For this review, take the finished solid that the model builds, in its own axes (mm). A direction names the side the tool comes from. Give positions to 0.01 mm unless a question says otherwise; leave off trailing zeros. Order: outer loops, then holes, each group sorted by start corner. A loop starts at its lowest first (then second) coordinate and runs counter-clockwise, first axis right, second up. Notation, with made-up numbers: (18.25, 63.5) - (41.25, 63.5) arc R15 ccw to (41.25, 86.5) - close; hole circle Ø1 at (63, -18.75). An arc over 180 degrees is marked (long way). Use a Markdown table: item, result. Add a question column.
1) We need section A-A on y = 5.5. Write out the cut boundary in (x, z), then the cut area to 3 significant figures.
2) We need section D-D on x = 15.25. Give the number of separate pieces and of enclosed holes in the cut face, then the cut area to 3 significant figures.
3) Wall thickness on L1, parallel to Z at x = 2, y = -13.5; L2, parallel to X at y = 27, z = -15; L3, parallel to Y at x = 18.25, z = -12.5: over which ranges is each line inside the solid? List them lowest first.
4) Machinability: for faces 1 (the face through (20, -7.25, -11)), 2 (the face through (17, 0, -1)), 3 (the face through (23, 26, -12.95)), which of the approach directions +Z, -Z, +X, -X, +Y, -Y give a long, thin tool a straight path to every point of the face, cutting with its end or side? Answer none if there is none.
5) Mouldability with a two-part tool opening along Y and no side actions: class faces 4 (the face through (20, -6, -13.6)), 5 (the face through (20, -4.25, -11)), 6 (the face through (9.367, 35.797, -1.141)), 7 (the face through (9.63, 5.95, -21.13)) as released by +Y, released by -Y, zero draft, split by the parting line, or undercut.
6) We need section C-C on y = 26. Write out the cut boundary in (x, z), then the cut area to 3 significant figures.
7) Clearance check with flat-ended pins moving along their axes: P1, Ø5, axis at y = 23.5, z = -19.5, coming from the -X side; P2, Ø2, axis at x = 20.5, z = -10, coming from the -Y side; P3, Ø6, axis at y = -7.5, z = -9.5, coming from the +X side. State where each tip first meets the part, or that it passes through.
8) We need section B-B on z = -7.75. Write out the cut boundary in (x, y).
Autodesk Inventor part; units mm, degrees
ref_plane "YZ Plane" through (0, 0, 0) normal (1, 0, 0) x (0, 1, 0)
ref_plane "XZ Plane" through (0, 0, 0) normal (0, 1, 0) x (-1, 0, 0)
ref_plane "XY Plane" through (0, 0, 0) normal (0, 0, 1) x (1, 0, 0)
sketch "Sketch1" plane through (0, 0, 0) normal (1, 0, 0) x (0, 1, 0)
  line L0 (0, 0) -> (33, 0)
  line L1 (37, -4) -> (37, -18.2)
  line L2 (33, -22.2) -> (0, -22.2)
  line L3 (0, -22.2) -> (0, 0)
  arc A0 (33, -22.2) -> (37, -18.2) centre (33, -18.2) ccw
  arc A1 (37, -4) -> (33, 0) centre (33, -4) ccw
extrude "Extrusion1" add sketch "Sketch1" along normal blind 19
sketch "Sketch2" plane through (19, 0, 0) normal (1, 0, 0) x (0, 0, -1)
  line L0 (0, 33) -> (0, 0)
  line L1 (22.2, 37) -> (0, 37)
  line L2 (0, 37) -> (0, 26)
  line L3 (22.2, 26) -> (22.2, 37)
  line L4 (0, 31.5) -> (0, 26)
  circle A0 centre (11.1, 26) radius 2.65
  dimension "d9" = 11
  dimension "d11" = 5.3
extrude "Extrusion2" add sketch "Sketch2" along normal blind 8
sketch "Sketch3" plane through (27, 26, -11.1) normal (1, 0, 0) x (0, 0, -1)
  line L0 (1.85, 0) -> (1.85, -3.8405)
  line L1 (1.85, -3.8405) -> (0, -3.8405)
  line L2 (1.85, -3.8405) -> (-1.85, -3.8405)
  line L3 (-1.85, -3.8405) -> (-1.85, 4.0175)
  line L4 (-1.85, 4.0175) -> (1.85, 4.0175)
  line L5 (1.85, 4.0175) -> (1.85, -3.8405)
  line L6 (1.85, 4.0175) -> (3.7589, 4.0175)
  line L7 (3.7589, 4.0175) -> (3.7589, -3.8405)
  line L8 (3.7589, -3.8405) -> (1.85, -3.8405)
  line L9 (1.85, -3.8405) -> (1.85, 4.0175)
  line L10 (-1.85, 4.0175) -> (-3.5435, 4.0175)
  line L11 (-3.5435, 4.0175) -> (-3.5435, -3.8405)
  line L12 (-3.5435, -3.8405) -> (-1.85, -3.8405)
  line L13 (-1.85, -3.8405) -> (-1.85, 4.0175)
  point P0 (-11.1, -26)
  dimension "d14" = 1.85
  dimension "d15" = 3.7
extrude "Extrusion3" cut sketch "Sketch3" against normal blind 8 contours L5 L6 L7 L8 L0 | L3 L12 L11 L10
sketch "Sketch4" plane through (19, 0, 0) normal (1, 0, 0) x (0, 0, -1)
  line L0 (0, 0) -> (22.2, 0)
  line L1 (0, 0) -> (22.2, 0)
  line L2 (22.2, 0) -> (22.2, 5.5)
  line L3 (0, 5.5) -> (0, 0)
  circle A0 centre (2.5, 5.5) radius 1.5
  circle A1 centre (19.7, 5.5) radius 1.5
  dimension "d18" = 5.5
  dimension "d20" = 3
  dimension "d22" = 3
extrude "Extrusion4" cut sketch "Sketch4" against normal blind 20
sketch "Sketch5" plane through (0, 0, -22.2) normal (0, -1, 0) x (1, 0, 0)
  line L0 (0, 22.2) -> (19, 22.2)
  line L1 (0, 0) -> (19, 0)
  line L2 (19, 18.2) -> (19, 22.2)
  line L3 (19, 22.2) -> (10, 22.2)
  line L4 (18, 0) -> (19, 0)
  line L5 (19, 4.6031) -> (19, 17.5969)
  line L6 (0.8056, 17.3188) -> (0.8056, 4.8812)
  arc A0 (0.8056, 4.8812) -> (19, 4.6031) centre (10, 11.1) ccw
  arc A1 (19, 17.5969) -> (0.8056, 17.3188) centre (10, 11.1) ccw
  arc A2 (1.8056, 5.1956) -> (18, 4.9348) centre (10, 11.1) ccw
  arc A3 (18, 17.2652) -> (1.8056, 17.0044) centre (10, 11.1) ccw
  line L7 (1.8056, 17.0044) -> (1.8056, 5.1956)
  line L8 (0.8056, 4.8812) -> (0.8056, 17.3188)
  line L9 (18, 17.2652) -> (18, 4.9348)
  line L10 (19, 4.6031) -> (19, 17.5969)
extrude "Extrusion5" add sketch "Sketch5" along normal blind 11.5
sketch "Sketch6" plane through (18, 0, -17.2652) normal (0, -1, 0) x (1, 0, 0)
  line L0 (-16.1944, 12.0697) -> (-16.1944, 0.2608)
  arc A0 (-16.1944, 0.2608) -> (0, 0) centre (-8, 6.1652) ccw
  line L1 (0, 0) -> (0, 12.3305)
  arc A1 (0, 12.3305) -> (-16.1944, 12.0697) centre (-8, 6.1652) ccw
  line L2 (-16.1944, 12.0697) -> (-16.1944, 0.2608)
  arc A2 (-16.1944, 0.2608) -> (0, 0) centre (-8, 6.1652) ccw
  line L3 (0, 0) -> (0, 12.3305)
  arc A3 (0, 12.3305) -> (-16.1944, 12.0697) centre (-8, 6.1652) ccw
  point P0 (-18, 17.2652)
extrude "Extrusion6" add sketch "Sketch6" along normal blind 25
fillet "Fillet1" radius 2 4 edges at (18, -25, -11.1) (9.8374, -25, -21.1987) (1.8056, -25, -11.1) (9.8374, -25, -1.0013)
sketch "Sketch7" plane through (19, 0, 0) normal (1, 0, 0) x (0, 0, -1)
  line L0 (4.6031, 0) -> (4.6031, -11.5)
  line L1 (17.5969, 0) -> (17.5969, -11.5)
  line L2 (22.2, 0) -> (0, 0)
  line L3 (13.6, -4.25) -> (8.6, -4.25)
  line L4 (8.6, -4.25) -> (8.6, -7.25)
  line L5 (8.6, -7.25) -> (13.6, -7.25)
  line L6 (13.6, -7.25) -> (13.6, -4.25)
  line L7 (13.6, -4.25) -> (8.6, -7.25) construction
  line L8 (8.6, -4.25) -> (13.6, -7.25) construction
  dimension "d33" = 5
  dimension "d34" = 3
extrude "Extrusion7" add sketch "Sketch7" along normal blind 2
sketch "Sketch8" plane through (0.8056, 0, -17.3188) normal (-1, 0, 0) x (0, 0, 1)
  line L0 (-4.8812, 0) -> (17.3188, 0)
  line L1 (3.7188, -4.25) -> (3.7188, -7.25)
  line L2 (8.7188, -7.25) -> (3.7188, -7.25)
  line L3 (3.7188, -7.25) -> (3.7188, -4.25)
  line L4 (3.7188, -4.25) -> (8.7188, -4.25)
  line L5 (8.7188, -4.25) -> (8.7188, -7.25)
  line L6 (8.7188, -7.25) -> (3.7188, -4.25) construction
  line L7 (3.7188, -7.25) -> (8.7188, -4.25) construction
  point P0 (6.2188, -5.75)
extrude "Extrusion8" add sketch "Sketch8" along normal blind 2
scale "Scale1" factors (2, 2, 2) then translate (-19, -12.75, 11.1) bodies 1
scale "Scale2" factors (0.5, 0.5, 0.5) then translate (9.5, 6.375, -5.55) bodies 1
properties part number "DCMotor"
Checked values:
| question | item | result |
|---|---|---|
| 1 | outline | (0, -22.2) - (19, -22.2) - (19, -21.2) - (0, -21.2) - close; (0, -18.2) - (19, -18.2) - (19, -4) - (0, -4) - close; (0, -1) - (19, -1) - (19, 0) - (0, 0) - close |
| 1 | area | 308 mm² |
| 2 | separate pieces | 1 |
| 2 | enclosed holes | 2 |
| 2 | area | 1,260 mm² |
| 3 | L1 | -17.27 to -4.93 |
| 3 | L2 | 0 to 19 |
| 3 | L3 | -11.5 to 37 |
| 4 | face 1 | +Z, -Z, +X, -Y |
| 4 | face 2 | +Z, +X, -Y |
| 4 | face 3 | -Z, +X, +Y |
| 5 | face 4 | zero draft |
| 5 | face 5 | undercut |
| 5 | face 6 | released by +Y |
| 5 | face 7 | undercut |
| 6 | outline | (0, -22.2) - (19, -22.2) - (19, -12.95) - (27, -12.95) - (27, -9.25) - (19, -9.25) - (19, 0) - (0, 0) - close |
| 6 | area | 451 mm² |
| 7 | P1 | x = 0 |
| 7 | P2 | y = -7.25 |
| 7 | P3 | x = 21 |
| 8 | outline | (0, 0) - (0.81, 0) - (0.81, -11.5) - (1.81, -11.5) - (1.81, -23) arc R2 ccw to (3.81, -25) - (16, -25) arc R2 ccw to (18, -23) - (18, -11.5) - (19, -11.5) - (19, 37) - (0, 37) - close |
